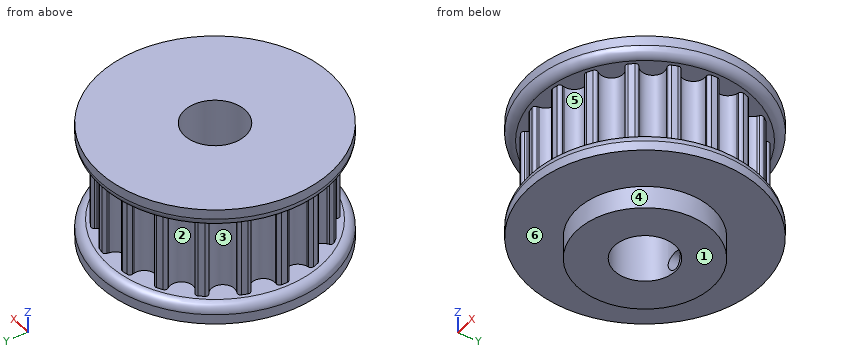
from build123d import *

# Parameters (mm, degrees)
SKETCH_3_R                       = 13.752444878
EXTRUDE_2_DEPTH                  = 5.5
CUT_EXTRUDE_2_DEPTH              = 21.211617458
FILLET_1_R                       = 0.4
PATTERN_CIRCULAR_1_COUNT         = 18
FILLET_1_OF_PATTERN_CIRCULAR_1_R = 0.4
SKETCH_12_R                      = 15.452444878
EXTRUDE_4_DEPTH                  = 2.5
EXTRUDE_START                    = 2.5
SKETCH_13_R                      = 15.452444878
EXTRUDE_5_DEPTH                  = 2.5
FILLET_2_R                       = 1.2
SKETCH_5_R                       = 9
EXTRUDE_3_DEPTH                  = 3
SKETCH_4_R                       = 4.05
CUT_EXTRUDE_3_DEPTH              = 29.957833284
SKETCH_8_W                       = 1.2
SKETCH_8_H                       = 15.452444878


with BuildPart() as part:
    # Sketch 3 → Extrude 2 (new, symmetric)
    with BuildSketch(Plane.XY):
        Circle(SKETCH_3_R)
    extrude(amount=EXTRUDE_2_DEPTH, both=True)

    # Sketch 3_3 → Cut-Extrude 2 (cut, symmetric)
    with BuildSketch(Plane.XY):
        with BuildLine():
            Line((-1.600765204, 13.658963756), (-1.524565963, 13.008773041))
            ThreePointArc((-1.524565963, 13.008773041), (0, 11.652444878), (1.524565963, 13.008773041))
            Line((1.524565963, 13.008773041), (1.600765204, 13.658963756))
            ThreePointArc((1.600765204, 13.658963756), (0, 13.752444878), (-1.600765204, 13.658963756))
        make_face()
    cut_extrude_2 = extrude(amount=CUT_EXTRUDE_2_DEPTH, both=True, mode=Mode.SUBTRACT)

    # Fillet 1
    fillet_1_edges = [part.edges().sort_by_distance(p)[0] for p in [
        (-1.600765204, 13.658963756, 0),
        (1.600765204, 13.658963756, 0),
    ]]
    fillet(fillet_1_edges, radius=FILLET_1_R)

    # Pattern Circular 1: Cut-Extrude 2 ×18 about axis
    pattern_circular_1_axis = Axis((0, 0, 0), (0, 0, 1))
    for i in range(1, PATTERN_CIRCULAR_1_COUNT):
        add(cut_extrude_2.rotate(pattern_circular_1_axis, i * 360 / PATTERN_CIRCULAR_1_COUNT), mode=Mode.SUBTRACT)

    # Fillet 1 of Pattern Circular 1
    fillet_1_of_pattern_circular_1_edges = [part.edges().sort_by_distance(p)[0] for p in [
        (-6.175867991, 12.287733505, 0),
        (-3.167413492, 13.382721394, 0),
        (-10.006069953, 9.434421245, 0),
        (-7.553555375, 11.492325323, 0),
        (-12.629392204, 5.443178546, 0),
        (-11.028627, 8.21578521, 0),
        (-13.729423366, 0.795408182, 0),
        (-13.173483445, 3.948300149, 0),
        (-13.173483445, -3.948300149, 0),
        (-13.729423366, -0.795408182, 0),
        (-11.028627, -8.21578521, 0),
        (-12.629392204, -5.443178546, 0),
        (-7.553555375, -11.492325323, 0),
        (-10.006069953, -9.434421245, 0),
        (-3.167413492, -13.382721394, 0),
        (-6.175867991, -12.287733505, 0),
        (1.600765204, -13.658963756, 0),
        (-1.600765204, -13.658963756, 0),
        (6.175867991, -12.287733505, 0),
        (3.167413492, -13.382721394, 0),
        (10.006069953, -9.434421245, 0),
        (7.553555375, -11.492325323, 0),
        (12.629392204, -5.443178546, 0),
        (11.028627, -8.21578521, 0),
        (13.729423366, -0.795408182, 0),
        (13.173483445, -3.948300149, 0),
        (13.173483445, 3.948300149, 0),
        (13.729423366, 0.795408182, 0),
        (11.028627, 8.21578521, 0),
        (12.629392204, 5.443178546, 0),
        (7.553555375, 11.492325323, 0),
        (10.006069953, 9.434421245, 0),
        (3.167413492, 13.382721394, 0),
        (6.175867991, 12.287733505, 0),
    ]]
    fillet(fillet_1_of_pattern_circular_1_edges, radius=FILLET_1_OF_PATTERN_CIRCULAR_1_R)

    # Sketch 12 → Extrude 4 (add)
    with BuildSketch(Plane.XY.offset(5.5)):
        Circle(SKETCH_12_R)
    extrude(amount=EXTRUDE_4_DEPTH)

    # Sketch 13 → Extrude 5 (add)
    with BuildSketch(Plane(origin=(0, 0, -5.5), x_dir=(-1, 0, 0), z_dir=(0, 0, -1)).offset(EXTRUDE_START)):
        with Locations(Location((0, 0, 0), (0, 0, 180))):
            Circle(SKETCH_13_R)
    extrude(amount=-EXTRUDE_5_DEPTH)

    # Fillet 2
    fillet_2_edges = [part.edges().sort_by_distance(p)[0] for p in [
        (-15.452444878, 0, 5.5),
        (-15.452444878, 0, -5.5),
    ]]
    fillet(fillet_2_edges, radius=FILLET_2_R)

    # Sketch 5 → Extrude 3 (add)
    with BuildSketch(Plane(origin=(0, 0, -8), x_dir=(-1, 0, 0), z_dir=(0, 0, -1))):
        Circle(SKETCH_5_R)
    extrude(amount=EXTRUDE_3_DEPTH)

    # Sketch 4 → Cut-Extrude 3 (cut, through all)
    with BuildSketch(Plane(origin=(0, 0, 8), x_dir=(-1, 0, 0), z_dir=(0, 0, -1))):
        Circle(SKETCH_4_R)
    extrude(amount=CUT_EXTRUDE_3_DEPTH, mode=Mode.SUBTRACT)

    # Sketch 8 → M3x0.5 _ _ _ _1 (revolve, cut)
    with BuildSketch(Plane(origin=(0, 0, -9.5), x_dir=(0, 0, -1), z_dir=(1, 0, 0))):
        with Locations((0.6, 7.726222439)):
            Rectangle(SKETCH_8_W, SKETCH_8_H)
    revolve(axis=Axis((0, -6.35, -9.5), (0, 1, 0)), mode=Mode.SUBTRACT)


solid = part.part
Here's how the part is built. I have some questions about the finished solid (model axes, mm). Face numbers are marked on the shaded views. A direction names the side the tool comes from. Round coordinates to 2 decimals unless told otherwise and drop trailing zeros. Order: outer loops, then holes, each group sorted by start corner. A loop starts at its lowest first (then second) coordinate and runs counter-clockwise, first axis right, second up. Notation, with made-up numbers: M -8.5,77 L 38.5,77 A23 cw 38.5,102 Z; hole C 43,0.25 d10. An arc over 180 degrees is marked long. Return JSON: item names as keys, results as strings. Group by question number.
1. If we section it at B-B on x = 0: List the corners of the cut face in (y, z) for me.
2. Please list where these lines run through material, in increasing order: probe 1 along Z at (x, y) = (-5, 13.5); probe 2 along Y at (x, z) = (10.5, 0); probe 3 along X at (y, z) = (0, -2.5).
3. If we mould it in two halves opening along X, with no side actions, what happens to the marked faces 3, 4, 5 and 6? For each: pulls with the +X half, pulls with the -X half, needs draft (parallel to the pull), parting line crosses it, or undercut.
4. On a 3-axis mill with a long thin cutter (end or side, diameter ignored), from which of +Z, -Z, +X, -X, +Y, -Y can I reach the whole of each face in a straight line? I mean the marked faces 1 and 2. Say none if no direction works.
5. I'm going to push flat-ended pins straight in: pin 1 Ø8 at (y, z) = (-9, -3) entering from +X; pin 2 Ø1 at (y, z) = (5, 5.5) entering from -X; pin 3 Ø1 at (x, z) = (9.5, -1) entering from +Y. Where does each tip first touch, or does it pass through?
6. If we section it at A-A on y = 0: List the corners of the cut face in (x, z) for me.
7. If we section it at C-C on z = -9.5: List the corners of the cut face in (x, y) for me, then the cut area to 3 significant figures.
Reply:
{
 "1": {"outline": "M -15.45,-8 L -9,-8 L -9,-11 L -4.05,-11 L -4.05,8 L -15.45,8 L -15.45,6.7 A1.2 ccw -14.25,5.5 L -11.65,5.5 L -11.65,-5.5 L -14.25,-5.5 A1.2 ccw -15.45,-6.7 Z; M 4.05,-11 L 9,-11 L 9,-10.7 L 4.05,-10.7 Z; M 4.05,-8.3 L 9,-8.3 L 9,-8 L 15.45,-8 L 15.45,-6.7 A1.2 ccw 14.25,-5.5 L 11.65,-5.5 L 11.65,5.5 L 14.25,5.5 A1.2 ccw 15.45,6.7 L 15.45,8 L 4.05,8 Z"},
 "2": {"probe 1": "-8 to -5.51, 5.51 to 8", "probe 2": "-8.88 to -7.82, -5.37 to 5.37, 7.82 to 8.88", "probe 3": "-13.75 to -4.05, 4.05 to 13.75"},
 "3": {"face 3": "undercut", "face 4": "parting line crosses it", "face 5": "undercut", "face 6": "needs draft"},
 "4": {"face 1": "-Z, +X, -X, +Y, -Y", "face 2": "none"},
 "5": {"pin 1": "x = 13.86", "pin 2": "x = -14.42", "pin 3": "y = 9.26"},
 "6": {"outline": "M -15.45,-8 L -9,-8 L -9,-11 L -4.05,-11 L -4.05,8 L -15.45,8 L -15.45,6.7 A1.2 ccw -14.25,5.5 L -13.75,5.5 L -13.75,-5.5 L -14.25,-5.5 A1.2 ccw -15.45,-6.7 Z; M 4.05,-11 L 9,-11 L 9,-8 L 15.45,-8 L 15.45,-6.7 A1.2 ccw 14.25,-5.5 L 13.75,-5.5 L 13.75,5.5 L 14.25,5.5 A1.2 ccw 15.45,6.7 L 15.45,8 L 4.05,8 Z"},
 "7": {"outline": "M -1.2,3.87 L -1.2,8.92 A9 ccw long 1.2,8.92 L 1.2,3.87 A4.05 cw long Z", "area": "191 mm^2"}
}
